Geometry: final body of the model. Coordinates: model frame, mm. A direction names the side the tool comes from. Give positions to 0.01 mm unless a question says otherwise; leave off trailing zeros. Loops run counter-clockwise (first coordinate to the right, second up) from the corner with the lowest first, then second, coordinate; pieces in that order, holes last. Notation, with made-up numbers: (-27, 87) - (32, 87) arc R18 ccw to (32, 100) - close; hole circle Ø9 at (15.5, 37). An arc over 180 degrees is marked (long way). Use one line per item in the form item = value.
Autodesk Inventor part; units mm, degrees
ref_plane "YZ Plane" through (0, 0, 0) normal (1, 0, 0) x (0, 1, 0)
ref_plane "XZ Plane" through (0, 0, 0) normal (0, 1, 0) x (-1, 0, 0)
ref_plane "XY Plane" through (0, 0, 0) normal (0, 0, 1) x (1, 0, 0)
ref_plane "작업 평면1" through (0, 0, 0) normal (0, 0, 1) x (1, 0, 0)
sketch "스케치1" plane through (0, 0, 0) normal (0, 0, 1) x (1, 0, 0)
  line L0 (0, 0) -> (6, 0)
  line L1 (6, 0) -> (6, 35)
  line L2 (0, 35) -> (6, 35)
  line L3 (0, 0) -> (0, 35)
  line L4 (0, 35) -> (70, 35)
  line L5 (70, 35) -> (70, 0)
  line L6 (70, 0) -> (0, 0)
  line L7 (0, 0) -> (0, 35)
  dimension "d4" = 0
  dimension "d0" = 70
extrude "돌출1" add sketch "스케치1" along normal blind 6
sketch "스케치2" plane through (0, 0, 6) normal (0, 0, 1) x (1, 0, 0)
  circle A0 centre (39, 6.5) radius 1.25
  circle A1 centre (31, 6.5) radius 1.25
  line L0 (25, 3) -> (45, 3)
  line L1 (45, 3) -> (45, 10)
  line L2 (45, 10) -> (25, 10)
  line L3 (25, 10) -> (25, 3)
  point P0 (0, 0)
extrude "돌출2" cut sketch "스케치2" against normal blind 6 contours A0 | A1
sketch "스케치3" plane through (0, 0, 6) normal (0, 0, 1) x (1, 0, 0)
  circle A0 centre (56, 28.5) radius 1.25
  circle A1 centre (64, 28.5) radius 1.25
  circle A2 centre (56, 28.5) radius 1.25
  line L0 (50, 32) -> (70, 32)
  line L1 (70, 32) -> (70, 25)
  line L2 (70, 25) -> (50, 25)
  line L3 (50, 25) -> (50, 32)
  circle A3 centre (12.5, 27) radius 1.25
  line L4 (9, 32) -> (16, 32)
  line L5 (16, 22) -> (16, 32)
  line L6 (9, 22) -> (16, 22)
  line L7 (9, 32) -> (9, 22)
  point P0 (0, 0)
extrude "돌출3" cut sketch "스케치3" against normal blind 6 contours A0 | A1 | A3
sketch "스케치4" plane through (0, 0, 6) normal (0, 0, 1) x (1, 0, 0)
  line L0 (15, 14) -> (15, 21)
  arc A0 (17, 23) -> (15, 21) centre (17, 21) ccw
  line L1 (17, 23) -> (53, 23)
  arc A1 (55, 21) -> (53, 23) centre (53, 21) ccw
  line L2 (55, 21) -> (55, 14)
  arc A2 (53, 12) -> (55, 14) centre (53, 14) ccw
  line L3 (53, 12) -> (17, 12)
  arc A3 (15, 14) -> (17, 12) centre (17, 14) ccw
  circle A4 centre (64, 28.5) radius 1.25
  circle A5 centre (56, 28.5) radius 1.25
  circle A6 centre (14, 27) radius 1.25
  circle A7 centre (39, 6.5) radius 1.25
  circle A8 centre (31, 6.5) radius 1.25
  line L4 (0, 0) -> (70, 0)
  line L5 (70, 0) -> (70, 35)
  line L6 (70, 35) -> (0, 35)
  line L7 (0, 35) -> (0, 0)
  point P0 (0, 0)
extrude "돌출4" cut sketch "스케치4" against normal blind 6 contours L0 A0 L1 A1 L2 A2 L3 A3
properties part number "61" material "아크릴, 선명"
(1) Pull-direction query (Y, two-part tool) for faces 3 (the face through (35, 26, 6)), 4 (the face through (35, 0, 3)), 5 (the face through (31.577, 5.391, 3.042)); classes: released by +Y, released by -Y, zero draft, split by the parting line, or undercut.
Solution:
face_3 = zero draft
face_4 = released by -Y
face_5 = undercut
(2) Cut plane D-D (z = 2.9). Return the cut outline in (x, y), plus the area to 3 significant figures.
Solution:
outline = (0, 0) - (70, 0) - (70, 35) - (0, 35) - close; hole circle Ø2.5 at (12.5, 27); hole (15, 14) arc R2 ccw to (17, 12) - (53, 12) arc R2 ccw to (55, 14) - (55, 21) arc R2 ccw to (53, 23) - (17, 23) arc R2 ccw to (15, 21) - close; hole circle Ø2.5 at (31, 6.5); hole circle Ø2.5 at (39, 6.5); hole circle Ø2.5 at (56, 28.5); hole circle Ø2.5 at (64, 28.5)
area = 1,990 mm2
(3) Pin query (flat end, axial travel): P1, Ø2, axis at x = 39, y = 6.5, coming from the +Z side. Return the tip coordinate at first contact, or that it passes through.
Solution:
P1 = through
(4) Access query for faces 1 (the face through (15.57, 12.6, 3.04)), 2 (the face through (35, 26, 0)). Directions: +Z, -Z, +X, -X, +Y, -Y. A direction counts if a zero-diameter tool reaches every point of the face in a straight line with its end or side. Return the directions, or none.
Solution:
face_1 = +Z, -Z
face_2 = -Z, +X, -X, +Y, -Y
(5) Cut plane B-B (y = 6.5). Return the cut outline in (x, z), plus the area to 3 significant figures.
Solution:
outline = (0, 0) - (29.75, 0) - (29.75, 6) - (0, 6) - close; (32.25, 0) - (37.75, 0) - (37.75, 6) - (32.25, 6) - close; (40.25, 0) - (70, 0) - (70, 6) - (40.25, 6) - close
area = 390 mm2
(6) Cut plane C-C (y = 19). Return the cut outline in (x, z).
Solution:
outline = (0, 0) - (15, 0) - (15, 6) - (0, 6) - close; (55, 0) - (70, 0) - (70, 6) - (55, 6) - close
(7) Material intervals for L1, parallel to Y at x = 31, z = 3.6; L2, parallel to X at y = 5.5, z = 1.15; L3, parallel to Y at x = 12.5, z = 1.75, sorted ascending. Write a range as from..to.
Solution:
L1 = 0..5.25, 7.75..12, 23..35
L2 = 0..30.25, 31.75..38.25, 39.75..70
L3 = 0..25.75, 28.25..35
(8) Cut plane A-A (x = 12.5). Return the cut outline in (y, z), plus the area to 3 significant figures.
Solution:
outline = (0, 0) - (25.75, 0) - (25.75, 6) - (0, 6) - close; (28.25, 0) - (35, 0) - (35, 6) - (28.25, 6) - close
area = 195 mm2
